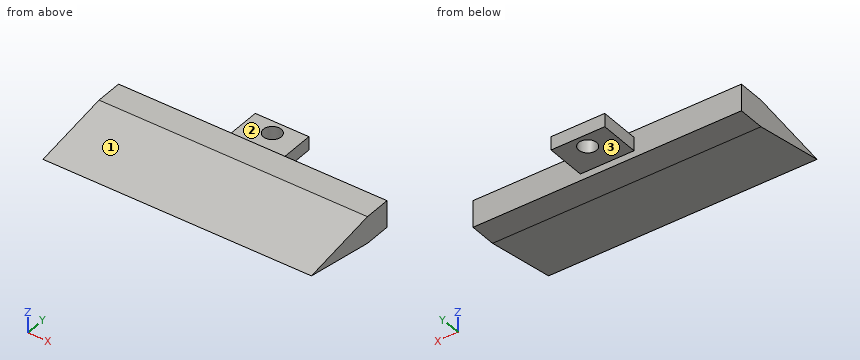
from build123d import *

# Parameters (mm, degrees)
BOSS_EXTRUDE1_DEPTH = 300
SKETCH2_W           = 60
SKETCH2_H           = 45
SKETCH2_R           = 10
BOSS_EXTRUDE2_DEPTH = 7.5


with BuildPart() as part:
    # Sketch1 → Boss-Extrude1 (new body)
    with BuildSketch(Plane(origin=(0, 0, 0), x_dir=(0, 0, -1), z_dir=(1, 0, 0))):
        Polygon((-15, 0), (15, 0), (15, -30), (0, -116), (-15, -30), align=None)
    extrude(amount=-BOSS_EXTRUDE1_DEPTH)

    # Sketch2 → Boss-Extrude2 (add, symmetric)
    with BuildSketch(Plane.XY):
        with Locations((-150, 22.5)):
            Rectangle(SKETCH2_W, SKETCH2_H)
        with Locations((-150, 30)):
            Circle(SKETCH2_R, mode=Mode.SUBTRACT)
    extrude(amount=BOSS_EXTRUDE2_DEPTH, both=True)


solid = part.part
The model under review builds one solid part; all positions refer to its coordinate system, in mm. Face numbers are marked on the shaded views. A direction names the side the tool comes from. Round coordinates to 2 decimals unless told otherwise and drop trailing zeros. Write each loop counter-clockwise with the first axis right and the second up, starting at its lowest first coordinate (ties: lowest second). Pieces come first, ordered by that corner, then holes. Notation, with made-up numbers: (10, 45) - (46, 45) arc R14 ccw to (46, 60) - close; hole circle Ø6 at (82, 60). An arc over 180 degrees is marked (long way). One line per item, written item: value. Start each with the question number.
1. To check wall thickness, follow L1, parallel to X at y = 16, z = 5.5; L2, parallel to Z at x = -41, y = -45; L3, parallel to Z at x = -194, y = -103. State the ranges of each line that lie inside material, in increasing order. Write a range as from..to.
2. Consider section D-D on x = -231. Write out the cut boundary in (y, z).
3. Consider section A-A on y = 30. Write out the cut boundary in (x, z).
4. Consider section C-C on z = 2.75. Write out the cut boundary in (x, y).
5. Machinability: for the marked faces 1, 2 and 3, which of the approach directions +Z, -Z, +X, -X, +Y, -Y give a long, thin tool a straight path to every point of the face, cutting with its end or side? Answer none if there is none.
6. Clearance check with flat-ended pins moving along their axes: P1, Ø7.5, axis at y = 16.5, z = -2.5, coming from the -X side; P2, Ø1, axis at x = -189.5, y = -44.5, coming from the -Z side; P3, Ø16.5, axis at y = 30.5, z = -2.5, coming from the +X side. State where each tip first meets the part, or that it passes through.
7. Consider section B-B on x = -150. Write out the cut boundary in (y, z).
Checks:
1. L1: x = -180..-120
1. L2: z = -12.38..12.38
1. L3: z = -2.27..2.27
2. outline: (-116, 0) - (-30, -15) - (0, -15) - (0, 15) - (-30, 15) - close
3. outline: (-180, -7.5) - (-160, -7.5) - (-160, 7.5) - (-180, 7.5) - close; (-140, -7.5) - (-120, -7.5) - (-120, 7.5) - (-140, 7.5) - close
4. outline: (-300, -100.23) - (0, -100.23) - (0, 0) - (-120, 0) - (-120, 45) - (-180, 45) - (-180, 0) - (-300, 0) - close; hole circle Ø20 at (-150, 30)
5. face 1: +Z, +X, -X, -Y
5. face 2: +Z, +X, -X, +Y
5. face 3: -Z, +X, -X, +Y
6. P1: stops at x = -180
6. P2: stops at z = -12.56
6. P3: stops at x = -120
7. outline: (-116, 0) - (-30, -15) - (0, -15) - (0, -7.5) - (20, -7.5) - (20, 7.5) - (0, 7.5) - (0, 15) - (-30, 15) - close; (40, -7.5) - (45, -7.5) - (45, 7.5) - (40, 7.5) - close
